Here's the drawing with two shaded views (mm, measured from the low corner). I have some questions. A direction names the side the tool comes from. Round coordinates to 2 decimals unless told otherwise and drop trailing zeros. Order: outer loops, then holes, each group sorted by start corner. A loop starts at its lowest first (then second) coordinate and runs counter-clockwise, first axis right, second up.
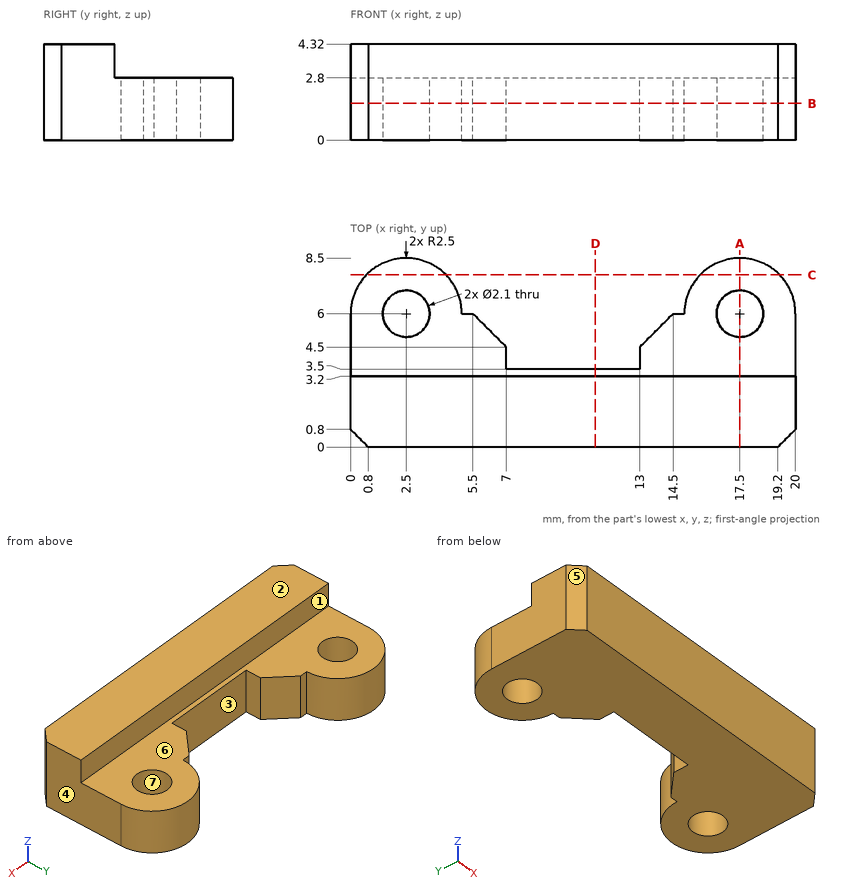
1. If we section it at C-C, the plane y = 7.75: Write out the boundary of the cut face in (x, z).
Evaluation:
outline: (0.71, 0) - (4.29, 0) - (4.29, 2.8) - (0.71, 2.8) - close; (15.71, 0) - (19.29, 0) - (19.29, 2.8) - (15.71, 2.8) - close
2. On a 3-axis mill with a long thin cutter (end or side, diameter ignored), from which of +Z, -Z, +X, -X, +Y, -Y can I reach the whole of each face in a straight line? I mean the marked faces 1, 2 and 3. Say none if no direction works.
Evaluation:
face 1: +Z, +X, -X, +Y
face 2: +Z, +X, -X, +Y, -Y
face 3: +Z, -Z, +Y
3. If we section it at A-A, the plane x = 17.5: Write out the boundary of the cut face in (y, z), and give its area (3 significant figures).
Evaluation:
outline: (0, 0) - (4.95, 0) - (4.95, 2.8) - (3.2, 2.8) - (3.2, 4.32) - (0, 4.32) - close; (7.05, 0) - (8.5, 0) - (8.5, 2.8) - (7.05, 2.8) - close
area: 22.8 mm2
4. I'm going to push flat-ended pins straight in: P1, Ø0.6, axis at x = 5, z = 1.5, coming from the +Y side; P2, Ø1.2, axis at x = 15, z = 3.5, coming from the +Y side; P3, Ø1.5, axis at x = 15.5, y = 6, coming from the +Z side; P4, Ø4, axis at x = 8.5, y = 7, coming from the +Z side. Where does each tip first touch, or does it pass through?
Evaluation:
P1: stops at y = 7.19
P2: stops at y = 3.2
P3: stops at z = 2.8
P4: passes through
5. I need wall thicknesses on probe 1 along Y at (x, z) = (17.5, 1.35); probe 2 along X at (y, z) = (5.75, 0.8); probe 3 along Z at (x, y) = (13.5, 3.25). Which ranges of each line are inside material? Lowest first, please.
Evaluation:
probe 1: y = 0 to 4.95, 7.05 to 8.5
probe 2: x = 0 to 1.48, 3.52 to 5.75, 14.25 to 16.48, 18.52 to 20
probe 3: z = 0 to 2.8
6. If we mould it in two halves opening along X, with no side actions, what happens to the marked faces 4, 5, 6 and 7? For each: released by +X, released by -X, zero draft, split by the parting line, or undercut.
Evaluation:
face 4: released by +X
face 5: released by -X
face 6: zero draft
face 7: undercut
7. If we section it at D-D, the plane x = 11: Write out the boundary of the cut face in (y, z).
Evaluation:
outline: (0, 0) - (3.5, 0) - (3.5, 2.8) - (3.2, 2.8) - (3.2, 4.32) - (0, 4.32) - close
8. If we section it at B-B, the plane z = 1.65: Write out the boundary of the cut face in (x, y).
Evaluation:
outline: (0, 0.8) - (0.8, 0) - (19.2, 0) - (20, 0.8) - (20, 6) arc R2.5 ccw to (15, 6) - (14.5, 6) - (13, 4.5) - (13, 3.5) - (7, 3.5) - (7, 4.5) - (5.5, 6) - (5, 6) arc R2.5 ccw to (0, 6) - close; hole circle Ø2.1 at (2.5, 6); hole circle Ø2.1 at (17.5, 6)
